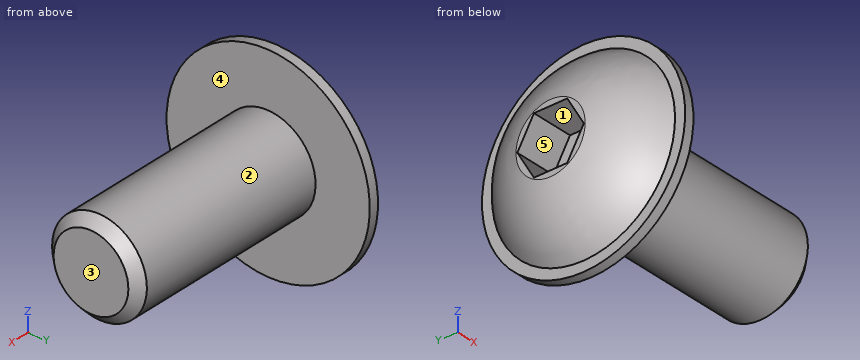
```python
from build123d import *

# Parameters (mm, degrees)
SKETCH2_R           = 3.96875
BOSS_EXTRUDE1_DEPTH = 17.4625
CUT_EXTRUDE1_DEPTH  = 3.556
CHAMFER1_SIZE       = 0.83947


with BuildPart() as part:
    # Sketch1 → Revolve1 (revolve)
    with BuildSketch(Plane.XY, mode=Mode.PRIVATE) as revolve1_sk:
        with BuildLine():
            Line((-4.064, 2.8956), (-4.064, 0))
            Line((-4.064, 0), (0, 0))
            Line((0, 0), (0, 8.509))
            Line((0, 8.509), (-0.8128, 8.509))
            Line((-0.8128, 8.509), (-0.8128, 7.6581))
            ThreePointArc((-0.8128, 7.6581), (-2.854131619, 5.560656119), (-4.064, 2.8956))
        make_face()
    revolve(revolve1_sk.sketch.rotate(Axis((-4.064, 0, 0), (1, 0, 0)), 270), axis=Axis((-4.064, 0, 0), (1, 0, 0)))

    # Sketch2 → Boss-Extrude1 (add)
    with BuildSketch(Plane(origin=(0, 0, 0), x_dir=(0, 0, -1), z_dir=(1, 0, 0))):
        Circle(SKETCH2_R)
    extrude(amount=BOSS_EXTRUDE1_DEPTH)

    # Sketch3 → Cut-Extrude1 (cut)
    with BuildSketch(Plane.ZY.offset(4.064)):
        Polygon((0, -2.786292399), (2.413, -1.3931462), (2.413, 1.3931462), (0, 2.786292399), (-2.413, 1.3931462), (-2.413, -1.3931462), align=None)
    extrude(amount=-CUT_EXTRUDE1_DEPTH, mode=Mode.SUBTRACT)

    # Chamfer1
    chamfer1_edges = [part.edges().sort_by_distance(p)[0] for p in [
        (17.4625, 0, 3.96875),
    ]]
    chamfer(chamfer1_edges, length=CHAMFER1_SIZE)


solid = part.part
```
Work out the finished part from the listing and answer in its coordinate system (mm). Face numbers are marked on the shaded views. A direction names the side the tool comes from. Round coordinates to 2 decimals unless told otherwise and drop trailing zeros. Write each loop counter-clockwise with the first axis right and the second up, starting at its lowest first coordinate (ties: lowest second). Pieces come first, ordered by that corner, then holes.
1) Determine the mould class of the marked faces 1, 2 and 3 for opening direction Y: pulls with the +Y half, pulls with the -Y half, needs draft (parallel to the pull), parting line crosses it, or undercut.
2) A cutting plane is placed at A-A on x = 6.25. Determine the outline of the cut face in (y, z).
3) Consider probe 1 along X at (y, z) = (0.5, 0.5); probe 2 along X at (y, z) = (2.25, 7.75); probe 3 along Z at (x, y) = (8.5, -0.5). Determine where each line is inside the solid, lowest interval first.
4) Which of the six approach directions +Z, -Z, +X, -X, +Y, -Y give full straight-line access (tool end or side, diameter ignored) to the marked faces 4 and 5?
5) Flat-ended cylindrical pins translate along their axes: P1, Ø1, axis at y = -5, z = -3, coming from the -X side; P2, Ø8, axis at x = 7, y = -3, coming from the -Z side; P3, Ø1.5, axis at x = 5, z = 2, coming from the -Y side; P4, Ø1, axis at x = 1.5, z = 5.5, coming from the -Y side. Find the tip coordinate at first contact, or state that the pin passes through.
Entries:
1. face 1: undercut
1. face 2: parting line crosses it
1. face 3: needs draft
2. outline: circle Ø7.94 at (0, 0)
3. probe 1: x = -0.51 to 17.46
3. probe 2: x = -0.81 to 0
3. probe 3: z = -3.94 to 3.94
4. face 4: +X
4. face 5: -X
5. P1: stops at x = -3.01
5. P2: stops at z = -3.97
5. P3: stops at y = -3.77
5. P4: passes through
